Design review of the part built by this model. Coordinates are the model's own, in mm. Give positions to 0.01 mm unless a question says otherwise; leave off trailing zeros. Loops run counter-clockwise (first coordinate to the right, second up) from the corner with the lowest first, then second, coordinate; pieces in that order, holes last. Notation, with made-up numbers: (55, -32.75) -> (111, -32.75) arc R11 cw to (111, -23.75) -> close; hole circle Ø4 at (43.25, 30). An arc over 180 degrees is marked (long way). Answer in a Markdown table with one row per item. Add a question column.
(1) For pin 1 (2.5 mm diameter, centred on x = 0, z = 13, fed in from +Y), flat-tipped, find the tip position at first contact; note if it passes through.
(2) Consider section C-C on z = 13. Write out the cut boundary in (x, y), then the cut area to 3 significant figures.
(3) Consider section B-B on y = -0.6. Write out the cut boundary in (x, z), then the cut area to 3 significant figures.
(4) Consider section A-A on x = 0. Write out the cut boundary in (y, z).
(5) Draft analysis for pull direction X (two halves, no side actions). For faces 1 (the cylindrical face through (-0.325, -1.528, -34.464)), 2 (the flat face through (0, -3.1, 1)), 3 (the flat face through (3, -2, 0)), state which applies: +X half, -X half, draft (parallel to the pull), parting line (faces both ways), or undercut.
(6) For line 1 (Z direction, x = 0, y = -2.05); line 2 (Z direction, x = 0.5, y = -1); line 3 (Z direction, x = 2.6, y = -2.45), list the stretches that pass through material, from the lowest coordinate up.
from build123d import *

# Parameters (mm, degrees)
F0_R     = 1.5
F1_DEPTH = 3.1


with BuildPart() as f1:
    # F0 (on Front) → F1 (new body)
    with BuildSketch(Plane.XZ):
        with BuildLine():
            Line((3, 0), (3, 33))
            ThreePointArc((3, 33), (0, 36), (-3, 33))
            Line((-3, 33), (-3, 0))
            Line((-3, 0), (-3, -33))
            ThreePointArc((-3, -33), (0, -36), (3, -33))
            Line((3, -33), (3, 0))
        make_face()
        with Locations((0, -33)):
            Circle(F0_R, mode=Mode.SUBTRACT)
        with Locations((0, 13)):
            Circle(F0_R, mode=Mode.SUBTRACT)
        with Locations((0, 33)):
            Circle(F0_R, mode=Mode.SUBTRACT)
    extrude(amount=F1_DEPTH)


solid = f1.part
Values follow:
| question | item | result |
|---|---|---|
| 1 | pin 1 | through |
| 2 | outline | (-3, -3.1) -> (-1.5, -3.1) -> (-1.5, 0) -> (-3, 0) -> close; (1.5, -3.1) -> (3, -3.1) -> (3, 0) -> (1.5, 0) -> close |
| 2 | area | 9.30 mm2 |
| 3 | outline | (-3, -33) arc R3 ccw to (3, -33) -> (3, 33) arc R3 ccw to (-3, 33) -> close; hole circle Ø3 at (0, -33); hole circle Ø3 at (0, 13); hole circle Ø3 at (0, 33) |
| 3 | area | 403 mm2 |
| 4 | outline | (-3.1, -36) -> (0, -36) -> (0, -34.5) -> (-3.1, -34.5) -> close; (-3.1, -31.5) -> (0, -31.5) -> (0, 11.5) -> (-3.1, 11.5) -> close; (-3.1, 14.5) -> (0, 14.5) -> (0, 31.5) -> (-3.1, 31.5) -> close; (-3.1, 34.5) -> (0, 34.5) -> (0, 36) -> (-3.1, 36) -> close |
| 5 | face 1 | undercut |
| 5 | face 2 | draft |
| 5 | face 3 | +X half |
| 6 | line 1 | -36 to -34.5, -31.5 to 11.5, 14.5 to 31.5, 34.5 to 36 |
| 6 | line 2 | -35.96 to -34.41, -31.59 to 11.59, 14.41 to 31.59, 34.41 to 35.96 |
| 6 | line 3 | -34.5 to 34.5 |
